from build123d import *

# Parameters (mm, degrees)
F3_DEPTH      = 38
F3_DEPTH_BACK = 10.001
F4_D          = 10.3


# Not quite as in the source:
# - an extrude ends at something that could not be found from the text; its depth is read off the source's solid


with BuildPart() as f2:
    # F1 (on Right) → F2 (revolve)
    with BuildSketch(Plane.YZ):
        Polygon((-10, 0), (0, 0), (0, 9.5), (-0.5349107164, 10.9696551146), (-9.4650892836, 10.9696551146), (-10, 9.5), align=None)
    revolve(axis=Axis((0, -5, 0), (0, -1, 0)))

    # F0 (on Front) → F3 (cut, two sides)
    with BuildSketch(Plane.XZ) as f3_sk:
        with BuildLine():
            Line((-9.5, 5.4848275573), (-4.7499997575, 8.227241476))
            Line((-4.7499997575, 8.227241476), (0, 10.9696551146))
            ThreePointArc((0, 10.9696551146), (-5.4848275573, 9.5), (-9.5, 5.4848275573))
        make_face()
        with BuildLine():
            Line((-9.5, -5.4848275573), (-9.5, 0))
            Line((-9.5, 0), (-9.5, 5.4848275573))
            ThreePointArc((-9.5, 5.4848275573), (-10.9696551146, 0), (-9.5, -5.4848275573))
        make_face()
        with BuildLine():
            Line((0, 10.9696551146), (4.7500001405, 8.2272412548))
            Line((4.7500001405, 8.2272412548), (9.5, 5.4848275573))
            ThreePointArc((9.5, 5.4848275573), (5.4848275573, 9.5), (0, 10.9696551146))
        make_face()
        with BuildLine():
            Line((9.5, 5.4848275573), (9.5, 0))
            Line((9.5, 0), (9.5, -5.4848275573))
            ThreePointArc((9.5, -5.4848275573), (10.5958731807, -2.8391556619), (10.9696551146, 0))
            ThreePointArc((10.9696551146, 0), (10.5958731807, 2.8391556619), (9.5, 5.4848275573))
        make_face()
        with BuildLine():
            Line((9.5, -5.4848275573), (4.7500001405, -8.2272412548))
            Line((4.7500001405, -8.2272412548), (0, -10.9696551146))
            ThreePointArc((0, -10.9696551146), (5.4848275573, -9.5), (9.5, -5.4848275573))
        make_face()
        with BuildLine():
            Line((0, -10.9696551146), (-4.7499999942, -8.2272413393))
            Line((-4.7499999942, -8.2272413393), (-9.5, -5.4848275573))
            ThreePointArc((-9.5, -5.4848275573), (-5.4848275573, -9.5), (0, -10.9696551146))
        make_face()
    extrude(amount=-F3_DEPTH, mode=Mode.SUBTRACT)
    extrude(f3_sk.sketch, amount=F3_DEPTH_BACK, mode=Mode.SUBTRACT)

    # F4 (through all)
    with Locations(Plane(origin=(0, 0, 0), x_dir=(1, 0, 0), z_dir=(0, 1, 0))):
        with Locations((0, 0)):
            Hole(F4_D / 2)


solid = f2.part
Work out the finished part from the listing and answer in its coordinate system (mm). Round coordinates to 2 decimals unless told otherwise and drop trailing zeros. Write each loop counter-clockwise with the first axis right and the second up, starting at its lowest first coordinate (ties: lowest second). Pieces come first, ordered by that corner, then holes.
1) Straight lines are drawn through the part: line 1 (Z direction, x = 2.75, y = -8.5); line 2 (X direction, y = -6.5, z = -3); line 3 (X direction, y = -2, z = 1). For each, find the intervals that lie inside material, in ascending order.
2) Given pin 1 Ø6 at (y, z) = (-2.5, -6) entering from -X; pin 2 Ø8 at (x, z) = (0, 0) entering from -Y, each flat-ended and moving along its own axis, determine where each tip first touches the part or whether it passes through.
3) A cutting plane is placed at A-A (y = -8.75). Give the vertices of the cut face in (x, z), plus the area to 3 significant figures.
4) The mould has two halves that part along X. Classify faces 1 (the cylindrical face through (-4.91, -5.07, -1.55)), 2 (the conical face through (-0.02, -0.13, -9.86)), 3 (the conical face through (-8.52, -0.13, 4.95)): pulls with the +X half, pulls with the -X half, needs draft (parallel to the pull), parting line crosses it, or undercut.
Completed:
1. line 1: z = -9.38 to -4.35, 4.35 to 9.38
1. line 2: x = -9.5 to -4.19, 4.19 to 9.5
1. line 3: x = -9.5 to -5.05, 5.05 to 9.5
2. pin 1: stops at x = -9.5
2. pin 2: passes through
3. outline: (-9.5, -5.48) - (0, -10.97) - (9.5, -5.48) - (9.5, 5.48) - (0, 10.97) - (-9.5, 5.48) - close; hole circle Ø10.3 at (0, 0)
3. area: 229 mm2
4. face 1: undercut
4. face 2: parting line crosses it
4. face 3: pulls with the -X half
